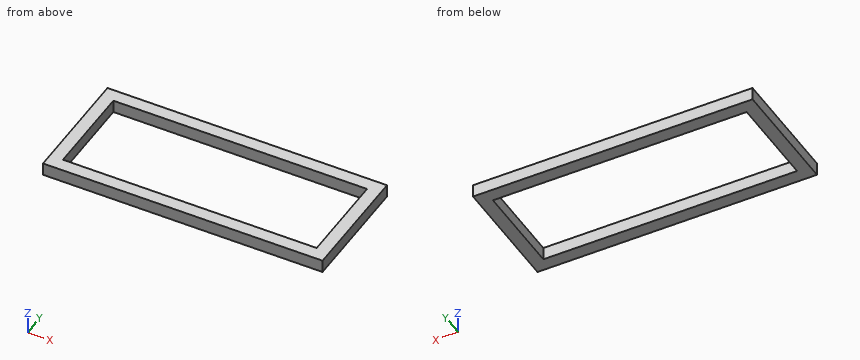
from build123d import *

# Parameters (mm, degrees)
F0_W     = 1300
F0_H     = 550
F0_W_2   = 1180
F0_H_2   = 430
F1_DEPTH = 30


with BuildPart() as f1:
    # F0 (on Top) → F1 (new body, symmetric)
    with BuildSketch(Plane.XY):
        with Locations((0, 303.536731)):
            Rectangle(F0_W, F0_H)
        with Locations((0, 303.536731)):
            Rectangle(F0_W_2, F0_H_2, mode=Mode.SUBTRACT)
    extrude(amount=F1_DEPTH, both=True)


solid = f1.part
Could you check a few things on this model? Use its own coordinates, in mm. Give positions to 0.01 mm unless a question says otherwise; leave off trailing zeros. Order: outer loops, then holes, each group sorted by start corner. A loop starts at its lowest first (then second) coordinate and runs counter-clockwise, first axis right, second up. Notation, with made-up numbers: (14, 54.5) - (39, 54.5) arc R7 ccw to (39, 61.5) - close; hole circle Ø9 at (-24, 59.5). An arc over 180 degrees is marked (long way). Return JSON: item names as keys, results as strings. Group by question number.
Q1. Please list where these lines run through material, in increasing order: line 1 along Y through (x, z) = (-585.5, -21); line 2 along X through (y, z) = (213, 12.5). Write a range as [from, to].
Q2. Suppose I cut it at C-C, the plane z = -6. Please give me the cut outline in (x, y), and give its area (3 significant figures).
Q3. Suppose I cut it at A-A, the plane y = 445. Please give me the cut outline in (x, z), and give its area (3 significant figures).
Q4. Suppose I cut it at B-B, the plane x = 144. Please give me the cut outline in (y, z), and give its area (3 significant figures).
Resolved:
{
 "1": {"line 1": "y = [28.54, 88.54], [518.54, 578.54]", "line 2": "x = [-650, -590], [590, 650]"},
 "2": {"outline": "(-650, 28.54) - (650, 28.54) - (650, 578.54) - (-650, 578.54) - close; hole (-590, 88.54) - (590, 88.54) - (590, 518.54) - (-590, 518.54) - close", "area": "208,000 mm2"},
 "3": {"outline": "(-650, -30) - (-590, -30) - (-590, 30) - (-650, 30) - close; (590, -30) - (650, -30) - (650, 30) - (590, 30) - close", "area": "7,200 mm2"},
 "4": {"outline": "(28.54, -30) - (88.54, -30) - (88.54, 30) - (28.54, 30) - close; (518.54, -30) - (578.54, -30) - (578.54, 30) - (518.54, 30) - close", "area": "7,200 mm2"}
}
